from build123d import *

# Parameters (mm, degrees)
CROQUIS1_W                   = 226
CROQUIS1_H                   = 45
SALIENTE_EXTRUIR1_DEPTH      = 6
CROQUIS2_W                   = 6
CROQUIS2_H                   = 30
SALIENTE_EXTRUIR2_DEPTH      = 6
SALIENTE_EXTRUIR2_DEPTH_BACK = 232


with BuildPart() as part:
    # Croquis1 → Saliente-Extruir1 (new body)
    with BuildSketch(Plane.XY):
        Rectangle(CROQUIS1_W, CROQUIS1_H)
    extrude(amount=SALIENTE_EXTRUIR1_DEPTH)

    # Croquis2 → Saliente-Extruir2 (add, two sides)
    with BuildSketch(Plane.ZY.offset(113)) as saliente_extruir2_sk:
        with Locations((3, 0)):
            Rectangle(CROQUIS2_W, CROQUIS2_H)
    extrude(amount=SALIENTE_EXTRUIR2_DEPTH)
    extrude(saliente_extruir2_sk.sketch, amount=-SALIENTE_EXTRUIR2_DEPTH_BACK)


solid = part.part
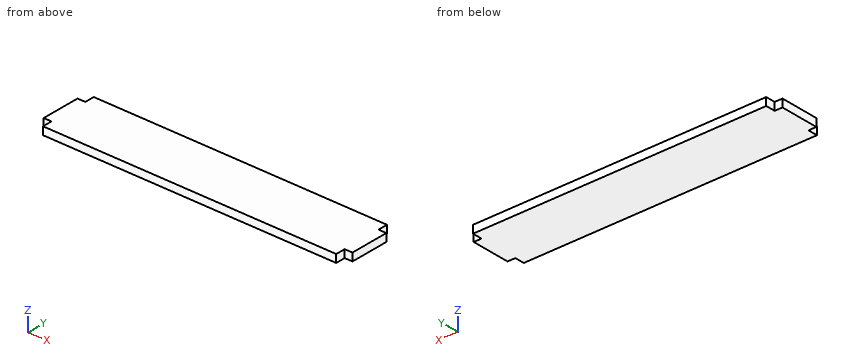
Check sheet for the modelled part. Datum: model origin and axes. Units: mm. Round coordinates to 2 decimals unless told otherwise and drop trailing zeros. Order: outer loops, then holes, each group sorted by start corner. A loop starts at its lowest first (then second) coordinate and runs counter-clockwise, first axis right, second up.
Q1. Cross-section at B-B, the plane y = -17.5. Enter the section's corners in (x, z), plus the area to 3 significant figures.
Filled sheet:
outline: (-113, 0) - (113, 0) - (113, 6) - (-113, 6) - close
area: 1,360 mm2
Q2. Depth check by flat-ended pin: P1, Ø3, axis at x = 115, z = 4.5, coming from the -Y side; P2, Ø1, axis at y = 16.5, z = 2.5, coming from the +X side. Enter the tip coordinate at first touch or a pass-through.
Filled sheet:
P1: stops at y = -15
P2: stops at x = 113
Q3. Cross-section at A-A, the plane z = 3.9. Enter the section's corners in (x, y), plus the area to 3 significant figures.
Filled sheet:
outline: (-119, -15) - (-113, -15) - (-113, -22.5) - (113, -22.5) - (113, -15) - (119, -15) - (119, 15) - (113, 15) - (113, 22.5) - (-113, 22.5) - (-113, 15) - (-119, 15) - close
area: 10,500 mm2
Q4. Scan line: L1, parallel to X at y = -16, z = 3.75. Record every from-to range of solid material in increasing order.
Filled sheet:
L1: x = -113 to 113
